Input: part model. Units: mm. Frame: model coordinates. Face numbers are marked on the shaded views. Round coordinates to 2 decimals unless told otherwise and drop trailing zeros. Loops run counter-clockwise (first coordinate to the right, second up) from the corner with the lowest first, then second, coordinate; pieces in that order, holes last.
(1) Draft query along Z for the marked faces 1, 2 and 3. Return one class per face: released by +Z, released by -Z, zero draft, split by the parting line, or undercut.
(2) Cut plane C-C, the plane z = -41.5. Output: boundary loops of the cut face in (x, y) (1 decimal).
(3) First-contact query: pin 1 Ø4 at (x, y) = (-40, 54) entering from -Z; pin 2 Ø3.5 at (x, z) = (13.89, 58.42) entering from -Y; pin 3 Ø3 at (x, z) = (-12.5, 0) entering from -Y; pin 4 Ø1.5 at (x, z) = (-26.5, -48.5) entering from -Y. Flat tips, straight axial feed; report the tip coordinate or a pass-through.
(4) Cut plane B-B, the plane y = 75.5. Output: boundary loops of the cut face in (x, z) (3 decimals).
(5) Cut plane A-A, the plane z = -28. Output: boundary loops of the cut face in (x, y) (1 decimal), and give its area (3 significant figures).
(6) Line query: line 1 (Y direction, x = -37.5, z = -29); line 2 (Y direction, x = 0, z = -7); line 3 (Z direction, x = 12.5, y = 110.8). Output: solid intervals per line, ascending.
from build123d import *

# Parameters (mm, degrees)
SKETCH1_R                      = 53.975
SKETCH1_R_2                    = 12.7
BOSS_EXTRUDE1_DEPTH            = 8.382
BOSS_EXTRUDE2_DEPTH            = 98.2345
SKETCH6_R                      = 53.975
SKETCH6_R_2                    = 6.55
BOSS_EXTRUDE6_DEPTH            = 4.8
CBORE_FOR_M3_SHCS1_D           = 3.3
CBORE_FOR_M3_SHCS1_DEPTH       = 4.8
CBORE_FOR_M3_SHCS1_CBORE_D     = 6.5
CBORE_FOR_M3_SHCS1_CBORE_DEPTH = 3
CUT_EXTRUDE2_DEPTH             = 129.229128673
BOSS_EXTRUDE7_START            = -4.8
SKETCH10_R                     = 2.3114
BOSS_EXTRUDE7_DEPTH            = 4.8
SKETCH11_W                     = 29.36875
SKETCH11_H                     = 96.079822772
CUT_EXTRUDE3_DEPTH             = 139.812722053


with BuildPart() as part:
    # Sketch1 → Boss-Extrude1 (new body)
    with BuildSketch(Plane(origin=(0, 0, 0), x_dir=(1, 0, 0), z_dir=(0, 1, 0))):
        with Locations(Location((0, 0, 0), (0, 0, 270))):
            Circle(SKETCH1_R)
        with Locations(Location((0, 0, 0), (0, 0, 270))):
            Circle(SKETCH1_R_2, mode=Mode.SUBTRACT)
    extrude(amount=BOSS_EXTRUDE1_DEPTH)

    # Sketch3 → Boss-Extrude2 (add)
    with BuildSketch(Plane(origin=(0, 8.382, 0), x_dir=(1, 0, 0), z_dir=(0, 1, 0))):
        with BuildLine():
            Line((13.49375, 45.673398559), (13.49375, 52.261069028))
            ThreePointArc((13.49375, 52.261069028), (-53.975, 0), (13.49375, -52.261069028))
            Line((13.49375, -52.261069028), (13.49375, -45.673398559))
            ThreePointArc((13.49375, -45.673398559), (-47.625, 0), (13.49375, 45.673398559))
        make_face()
    extrude(amount=BOSS_EXTRUDE2_DEPTH)

    # Sketch6 → Boss-Extrude6 (add)
    with BuildSketch(Plane(origin=(0, 106.6165, 0), x_dir=(1, 0, 0), z_dir=(0, 1, 0))):
        with Locations(Location((0, 0, 0), (0, 0, 270))):
            Circle(SKETCH6_R)
        with Locations(Location((0, 0, 0), (0, 0, 270))):
            Circle(SKETCH6_R_2, mode=Mode.SUBTRACT)
    extrude(amount=BOSS_EXTRUDE6_DEPTH)

    # CBORE for M3 SHCS1
    with Locations(Plane(origin=(0, 106.6165, 0), x_dir=(-1, 0, 0), z_dir=(0, -1, 0))):
        with Locations((-12.5, 0), (0, -12.5), (0, 12.5), (12.5, 0)):
            CounterBoreHole(CBORE_FOR_M3_SHCS1_D / 2, CBORE_FOR_M3_SHCS1_CBORE_D / 2, CBORE_FOR_M3_SHCS1_CBORE_DEPTH, depth=CBORE_FOR_M3_SHCS1_DEPTH)

    # Sketch3<3> → Cut-Extrude2 (cut, through all)
    with BuildSketch(Plane(origin=(0, 8.382, 0), x_dir=(1, 0, 0), z_dir=(0, 1, 0))):
        with BuildLine():
            ThreePointArc((13.49375, -52.261069028), (53.975, 0), (13.49375, 52.261069028))
            Line((13.49375, 52.261069028), (13.49375, 45.673398559))
            Line((13.49375, 45.673398559), (13.49375, -45.673398559))
            Line((13.49375, -45.673398559), (13.49375, -52.261069028))
        make_face()
    extrude(amount=-CUT_EXTRUDE2_DEPTH, mode=Mode.SUBTRACT)

    # Sketch10 → Boss-Extrude7 (add)
    with BuildSketch(Plane(origin=(0, 111.4165, 0), x_dir=(1, 0, 0), z_dir=(0, 1, 0)).offset(BOSS_EXTRUDE7_START)):
        with BuildLine():
            Line((-53.975, 58.42), (-53.975, 0))
            ThreePointArc((-53.975, 0), (-28.152959713, 46.051183311), (24.60625, 48.039911386))
            Line((24.60625, 48.039911386), (24.60625, 58.42))
            ThreePointArc((24.60625, 58.42), (23.327588042, 61.506963042), (20.240625, 62.785625))
            Line((20.240625, 62.785625), (-49.609375, 62.785625))
            ThreePointArc((-49.609375, 62.785625), (-52.696338042, 61.506963042), (-53.975, 58.42))
        make_face()
        with Locations(Location((-49.609375, 58.42, 0), (0, 0, 270))):
            Circle(SKETCH10_R, mode=Mode.SUBTRACT)
        with Locations(Location((-43.259375, 58.42, 0), (0, 0, 270))):
            Circle(SKETCH10_R, mode=Mode.SUBTRACT)
        with Locations(Location((-36.909375, 58.42, 0), (0, 0, 270))):
            Circle(SKETCH10_R, mode=Mode.SUBTRACT)
        with Locations(Location((-30.559375, 58.42, 0), (0, 0, 270))):
            Circle(SKETCH10_R, mode=Mode.SUBTRACT)
        with Locations(Location((-24.209375, 58.42, 0), (0, 0, 270))):
            Circle(SKETCH10_R, mode=Mode.SUBTRACT)
        with Locations(Location((-17.859375, 58.42, 0), (0, 0, 270))):
            Circle(SKETCH10_R, mode=Mode.SUBTRACT)
        with Locations(Location((-11.509375, 58.42, 0), (0, 0, 270))):
            Circle(SKETCH10_R, mode=Mode.SUBTRACT)
        with Locations(Location((-5.159375, 58.42, 0), (0, 0, 270))):
            Circle(SKETCH10_R, mode=Mode.SUBTRACT)
        with Locations(Location((1.190625, 58.42, 0), (0, 0, 270))):
            Circle(SKETCH10_R, mode=Mode.SUBTRACT)
        with Locations(Location((7.540625, 58.42, 0), (0, 0, 270))):
            Circle(SKETCH10_R, mode=Mode.SUBTRACT)
        with Locations(Location((13.890625, 58.42, 0), (0, 0, 270))):
            Circle(SKETCH10_R, mode=Mode.SUBTRACT)
        with Locations(Location((20.240625, 58.42, 0), (0, 0, 270))):
            Circle(SKETCH10_R, mode=Mode.SUBTRACT)
    boss_extrude7 = extrude(amount=BOSS_EXTRUDE7_DEPTH)

    # Mirror1: Boss-Extrude7 across plane
    add(boss_extrude7.mirror(Plane.XY))

    # Sketch11 → Cut-Extrude3 (cut, through all)
    with BuildSketch(Plane(origin=(0, 111.4165, 0), x_dir=(1, 0, 0), z_dir=(0, 1, 0))):
        with Locations((39.290625, 0)):
            Rectangle(SKETCH11_W, SKETCH11_H)
    extrude(amount=-CUT_EXTRUDE3_DEPTH, mode=Mode.SUBTRACT)


solid = part.part
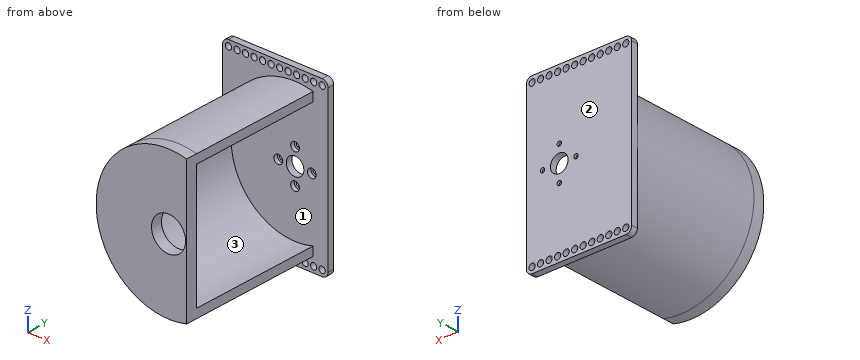
Reported:
1. face 1: undercut
1. face 2: zero draft
1. face 3: undercut
2. outline: (-54, 106.6) - (-34.5, 106.6) - (-34.5, 0) - (13.5, 0) - (13.5, 8.4) - (-23.4, 8.4) - (-23.4, 106.6) - (24.6, 106.6) - (24.6, 111.4) - (-54, 111.4) - close
3. pin 1: stops at z = -38.33
3. pin 2: passes through
3. pin 3: stops at y = 0
3. pin 4: stops at y = 106.62
4. outline: (13.494, -52.261) - (13.494, -45.673) arc R47.625 cw (long way) to (13.494, 45.673) - (13.494, 52.261) arc R53.975 ccw (long way) to start
5. outline: (-54, 106.6) - (-46.1, 106.6) - (-46.1, 0) - (13.5, 0) - (13.5, 8.4) - (-38.5, 8.4) - (-38.5, 106.6) - (24.6, 106.6) - (24.6, 111.4) - (-54, 111.4) - close
5. area: 1,630 mm2
6. line 1: y = 0 to 8.38, 106.62 to 111.42
6. line 2: y = 106.62 to 111.42
6. line 3: z = -62.79 to -60.27, -56.57 to -1.65, 1.65 to 56.57, 60.27 to 62.79
